Here's how the part is built. I have some questions about the finished solid (model axes, mm). A direction names the side the tool comes from. Round coordinates to 2 decimals unless told otherwise and drop trailing zeros. Order: outer loops, then holes, each group sorted by start corner. A loop starts at its lowest first (then second) coordinate and runs counter-clockwise, first axis right, second up. Notation, with made-up numbers: (-30.75, 58) - (-16.75, 58) arc R24 ccw to (-16.75, 86) - close; hole circle Ø1 at (74, 61). An arc over 180 degrees is marked (long way). Answer as a JSON object with one key per item and string values.
```python
from build123d import *

# Parameters (mm, degrees)
BOSS_EXTRUDE1_DEPTH = 6.3
BOSS_EXTRUDE2_DEPTH = 8
SKETCH3_R           = 3.5
CUT_EXTRUDE1_DEPTH  = 8
BOSS_EXTRUDE3_START = -8
BOSS_EXTRUDE3_DEPTH = 8
SKETCH5_W           = 30
SKETCH5_H           = 25
BOSS_EXTRUDE4_DEPTH = 8
FILLET1_R           = 10
BOSS_EXTRUDE5_START = 4.6
BOSS_EXTRUDE5_DEPTH = 4.6


with BuildPart() as part:
    # Sketch1 → Boss-Extrude1 (new body)
    with BuildSketch(Plane.XY):
        with BuildLine():
            Line((5, 4.5), (5, -4.5))
            ThreePointArc((5, -4.5), (0, -9.5), (-5, -4.5))
            Line((-5, -4.5), (-5, 4.5))
            ThreePointArc((-5, 4.5), (0, 9.5), (5, 4.5))
        make_face()
    extrude(amount=BOSS_EXTRUDE1_DEPTH)

    # Sketch2 → Boss-Extrude2 (add)
    with BuildSketch(Plane.XY.offset(6.3)):
        with BuildLine():
            Line((-4.5, 12.5), (4.5, 12.5))
            ThreePointArc((4.5, 12.5), (10.156854249, 10.156854249), (12.5, 4.5))
            Line((12.5, 4.5), (12.5, -4.5))
            ThreePointArc((12.5, -4.5), (10.156854249, -10.156854249), (4.5, -12.5))
            Line((4.5, -12.5), (-4.5, -12.5))
            ThreePointArc((-4.5, -12.5), (-10.156854249, -10.156854249), (-12.5, -4.5))
            Line((-12.5, -4.5), (-12.5, 4.5))
            ThreePointArc((-12.5, 4.5), (-10.156854249, 10.156854249), (-4.5, 12.5))
        make_face()
    extrude(amount=BOSS_EXTRUDE2_DEPTH)

    # Sketch3 → Cut-Extrude1 (cut)
    with BuildSketch(Plane.XY.offset(14.3)):
        Circle(SKETCH3_R)
    extrude(amount=-CUT_EXTRUDE1_DEPTH, mode=Mode.SUBTRACT)

    # Sketch4 → Boss-Extrude3 (add)
    with BuildSketch(Plane.XY.offset(14.3).offset(BOSS_EXTRUDE3_START)):
        with BuildLine():
            Line((-12.5, -4.5), (-12.5, -54.5))
            Line((-12.5, -54.5), (12.5, -54.5))
            Line((12.5, -54.5), (12.5, -4.5))
            ThreePointArc((12.5, -4.5), (10.156854249, -10.156854249), (4.5, -12.5))
            Line((4.5, -12.5), (-4.5, -12.5))
            ThreePointArc((-4.5, -12.5), (-10.156854249, -10.156854249), (-12.5, -4.5))
        make_face()
    extrude(amount=BOSS_EXTRUDE3_DEPTH)

    # Sketch5 → Boss-Extrude4 (add)
    with BuildSketch(Plane.XY.offset(14.3)):
        with Locations((-27.5, -42)):
            Rectangle(SKETCH5_W, SKETCH5_H)
    extrude(amount=-BOSS_EXTRUDE4_DEPTH)

    # Fillet1
    fillet1_edges = [part.edges().sort_by_distance(p)[0] for p in [
        (12.5, -54.5, 10.3),
        (-12.5, -29.5, 10.3),
        (-42.5, -54.5, 10.3),
        (-42.5, -29.5, 10.3),
    ]]
    fillet(fillet1_edges, radius=FILLET1_R)

    # Sketch6 → Boss-Extrude5 (add)
    with BuildSketch(Plane(origin=(0, 0, 6.3), x_dir=(-1, 0, 0), z_dir=(0, 0, -1)).offset(BOSS_EXTRUDE5_START)):
        with BuildLine():
            Line((-2.5, -19.5), (5.179491924, -19.5))
            ThreePointArc((5.179491924, -19.5), (10.179491924, -20.839745962), (13.839745962, -24.5))
            ThreePointArc((13.839745962, -24.5), (17.5, -28.160254038), (22.5, -29.5))
            Line((22.5, -29.5), (32.5, -29.5))
            ThreePointArc((32.5, -29.5), (39.571067812, -32.428932188), (42.5, -39.5))
            Line((42.5, -39.5), (42.5, -44.5))
            ThreePointArc((42.5, -44.5), (39.571067812, -51.571067812), (32.5, -54.5))
            Line((32.5, -54.5), (-2.5, -54.5))
            ThreePointArc((-2.5, -54.5), (-9.571067812, -51.571067812), (-12.5, -44.5))
            Line((-12.5, -44.5), (-12.5, -29.5))
            ThreePointArc((-12.5, -29.5), (-9.571067812, -22.428932188), (-2.5, -19.5))
        make_face()
    extrude(amount=-BOSS_EXTRUDE5_DEPTH)


solid = part.part
```
1. Imagine slicing it at D-D (y = -23). List the corners of the cut face in (x, z) for me, plus the area to 3 significant figures.
Responses:
{"outline": "(-13.13, 6.3) - (-12.78, 6.3) - (-12.78, 1.7) - (10.1, 1.7) - (10.1, 6.3) - (12.5, 6.3) - (12.5, 14.3) - (-13.13, 14.3) - close", "area": "310 mm2"}
2. Thinking about a two-plate mould opening in Y: for faces 5 (the face through (-4, -8, 6.3)), 6 (the face through (0.1, -9.5, 3.1)), 7 (the face through (0, 0, 0)), 8 (the face through (10.094, 10.219, 10.244)), which applies, pulls with the +Y half, pulls with the -Y half, needs draft (parallel to the pull), parting line crosses it, or undercut?
Responses:
{"face 5": "undercut", "face 6": "undercut", "face 7": "needs draft", "face 8": "pulls with the +Y half"}
3. Imagine slicing it at C-C (x = 0). List the corners of the cut face in (y, z) for me.
Responses:
{"outline": "(-54.5, 1.7) - (-19.5, 1.7) - (-19.5, 6.3) - (-9.5, 6.3) - (-9.5, 0) - (9.5, 0) - (9.5, 6.3) - (12.5, 6.3) - (12.5, 14.3) - (3.5, 14.3) - (3.5, 6.3) - (-3.5, 6.3) - (-3.5, 14.3) - (-54.5, 14.3) - close"}
4. For P1, Ø5, axis at y = 3, z = 8.5, coming from the -X side; P2, Ø1.4, axis at x = -0.5, z = 3.5, coming from the +Y side; P3, Ø8, axis at x = -29, z = 7, coming from the +Y side, each with a flat end and sliding along its axis, tell me the tip position at first contact or that it passes through.
Responses:
{"P1": "x = -12.5", "P2": "y = 9.5", "P3": "y = -29.5"}
5. For faces 1 (the face through (-15, -41, 1.7)), 2 (the face through (-27, -29.5, 8)), 3 (the face through (-1, -19.5, 4)), 4 (the face through (0, 0, 6.3)), which set-ups out of +Z, -Z, +X, -X, +Y, -Y let a thin tool reach every point of the face, with its end or its side?
Responses:
{"face 1": "-Z, +X, -X, -Y", "face 2": "+Z, -Z, -X, +Y", "face 3": "-Z, +X, -X", "face 4": "+Z"}
6. If I drill on L1, parallel to Y at x = 0, z = 11; L2, parallel to X at y = 4, z = 6.25; L3, parallel to Z at x = -0.5, y = 0, over which ranges is the centre line in solid material (lowest first)? Write a range as [from, to].
Responses:
{"L1": "[-54.5, -3.5], [3.5, 12.5]", "L2": "[-5, 5]", "L3": "[0, 6.3]"}
7. Imagine slicing it at B-B (z = 8.25). List the corners of the cut face in (x, y) for me, plus the area to 3 significant figures.
Responses:
{"outline": "(-42.5, -44.5) arc R10 ccw to (-32.5, -54.5) - (2.5, -54.5) arc R10 ccw to (12.5, -44.5) - (12.5, 4.5) arc R8 ccw to (4.5, 12.5) - (-4.5, 12.5) arc R8 ccw to (-12.5, 4.5) - (-12.5, -19.5) arc R10 cw to (-22.5, -29.5) - (-32.5, -29.5) arc R10 ccw to (-42.5, -39.5) - close; hole circle Ø7 at (0, 0)", "area": "2,320 mm2"}
8. Imagine slicing it at A-A (z = 3.5). List the corners of the cut face in (x, y) for me, plus the area to 3 significant figures.
Responses:
{"outline": "(-42.5, -44.5) arc R10 ccw to (-32.5, -54.5) - (2.5, -54.5) arc R10 ccw to (12.5, -44.5) - (12.5, -29.5) arc R10 ccw to (2.5, -19.5) - (-5.18, -19.5) arc R10 ccw to (-13.84, -24.5) arc R10 cw to (-22.5, -29.5) - (-32.5, -29.5) arc R10 ccw to (-42.5, -39.5) - close; (-5, -4.5) arc R5 ccw to (5, -4.5) - (5, 4.5) arc R5 ccw to (-5, 4.5) - close", "area": "1,720 mm2"}
